```python
from build123d import *

# Parameters (mm, degrees)
F1_DEPTH = 25.4


with BuildPart() as f1:
    # F0 (on Top) → F1 (new body)
    with BuildSketch(Plane.XY):
        with BuildLine():
            ThreePointArc((-16.6309525629, 0), (-25.9303122603, 22.4506403027), (-48.3809525629, 31.75))
            Line((-48.3809525629, 31.75), (-48.3809525629, 12.7))
            ThreePointArc((-48.3809525629, 12.7), (-39.4006964419, 8.9802561211), (-35.6809525629, 0))
            ThreePointArc((-35.6809525629, 0), (-39.4006964419, -8.9802561211), (-48.3809525629, -12.7))
            Line((-48.3809525629, -12.7), (-48.3809525629, -31.75))
            ThreePointArc((-48.3809525629, -31.75), (-25.9303122603, -22.4506403027), (-16.6309525629, 0))
        make_face()
        with BuildLine():
            Line((50.3968245514, 31.75), (-48.3809525629, 31.75))
            ThreePointArc((-48.3809525629, 31.75), (-25.9303122603, 22.4506403027), (-16.6309525629, 0))
            ThreePointArc((-16.6309525629, 0), (-25.9303122603, -22.4506403027), (-48.3809525629, -31.75))
            Line((-48.3809525629, -31.75), (50.3968245514, -31.75))
            Line((50.3968245514, -31.75), (50.3968245514, 31.75))
        make_face()
        with BuildLine():
            Line((-48.3809525629, 12.7), (-48.3809525629, 31.75))
            ThreePointArc((-48.3809525629, 31.75), (-80.1309525629, 0), (-48.3809525629, -31.75))
            Line((-48.3809525629, -31.75), (-48.3809525629, -12.7))
            ThreePointArc((-48.3809525629, -12.7), (-61.0809525629, 0), (-48.3809525629, 12.7))
        make_face()
    extrude(amount=F1_DEPTH)


solid = f1.part
```
Verification items for the finished model (mm, model axes). Give positions to 0.01 mm unless a question says otherwise; leave off trailing zeros. Write each loop counter-clockwise with the first axis right and the second up, starting at its lowest first coordinate (ties: lowest second). Pieces come first, ordered by that corner, then holes. Notation, with made-up numbers: M -12.5,80 L 6.5,80 A26 cw 6.5,100 Z; hole C -3,65 d7. An arc over 180 degrees is marked long. One line per question, with ' | ' between items.
1) Section check C-C on x = -53.5. Enter the section's corners in (y, z).
Result:
outline: M -31.33,0 L -11.62,0 L -11.62,25.4 L -31.33,25.4 Z; M 11.62,0 L 31.33,0 L 31.33,25.4 L 11.62,25.4 Z
2) Section check A-A on z = 15.5. Enter the section's corners in (x, y), plus the area to 3 significant figures.
Result:
outline: M -48.38,-31.75 L 50.4,-31.75 L 50.4,31.75 L -48.38,31.75 A31.75 ccw Z; hole C -48.38,0 d25.4 | area: 7,350 mm2
3) Thickness scan on line 1 along X through (y, z) = (-0.5, 5.75); line 2 along X through (y, z) = (6, 9.75); line 3 along Y through (x, z) = (-44.5, 2.75). Record the ranges inside material, lowest first. Write a range as [from, to].
Result:
line 1: x = [-80.13, -61.07], [-35.69, 50.4] | line 2: x = [-79.56, -59.57], [-37.19, 50.4] | line 3: y = [-31.75, -12.09], [12.09, 31.75]
4) Section check D-D on y = 25. Enter the section's corners in (x, z), plus the area to 3 significant figures.
Result:
outline: M -67.95,0 L 50.4,0 L 50.4,25.4 L -67.95,25.4 Z | area: 3,010 mm2
5) Section check B-B on x = -38. Enter the section's corners in (y, z).
Result:
outline: M -31.75,0 L -7.32,0 L -7.32,25.4 L -31.75,25.4 Z; M 7.32,0 L 31.75,0 L 31.75,25.4 L 7.32,25.4 Z
6) Gauge pin test, flat ends, axial feed: pin 1 Ø6 at (y, z) = (1, 14) entering from -X; pin 2 Ø12 at (x, y) = (-37, 11) entering from -Z. Record the tip position at first contact, or that the pin passes through.
Result:
pin 1: stops at x = -80.13 | pin 2: stops at z = 0
